Autodesk Inventor part; units mm, degrees
ref_plane "YZ Plane" through (0, 0, 0) normal (1, 0, 0) x (0, 1, 0)
ref_plane "XZ Plane" through (0, 0, 0) normal (0, 1, 0) x (-1, 0, 0)
ref_plane "XY Plane" through (0, 0, 0) normal (0, 0, 1) x (1, 0, 0)
sketch "Sketch1" plane through (0, 0, 0) normal (0, 1, 0) x (-1, 0, 0)
  line L0 (-3, 0) -> (-1.5, 2.5981)
  line L1 (-1.5, 2.5981) -> (1.5, 2.5981)
  line L2 (1.5, 2.5981) -> (3, 0)
  line L3 (3, 0) -> (1.5, -2.5981)
  line L4 (1.5, -2.5981) -> (-1.5, -2.5981)
  line L5 (-1.5, -2.5981) -> (-3, 0)
  point P0 (0, 0)
  point P1 (0, 0)
  dimension "d0" = 6
sketch "Sketch2" plane through (0, 0, 0) normal (0, 1, 0) x (-1, 0, 0)
  point P0 (0, 0)
extrude "Extrusion1" add sketch "Sketch1" along normal blind 25
sketch "Sketch3" plane through (0, 0, 0) normal (0, -1, 0) x (1, 0, 0)
  circle A0 centre (0, 0) radius 1.5
  dimension "d3" = 3
sketch "Sketch4" plane through (0, 25, 0) normal (0, 1, 0) x (1, 0, 0)
  circle A0 centre (0, 0) radius 1.5
  dimension "d4" = 3
extrude "Extrusion2" add sketch "Sketch3" along normal blind 8
extrude "Extrusion3" cut sketch "Sketch4" against normal blind 10
properties part number "Spacer25mm" material "Brass, Soft Yellow"
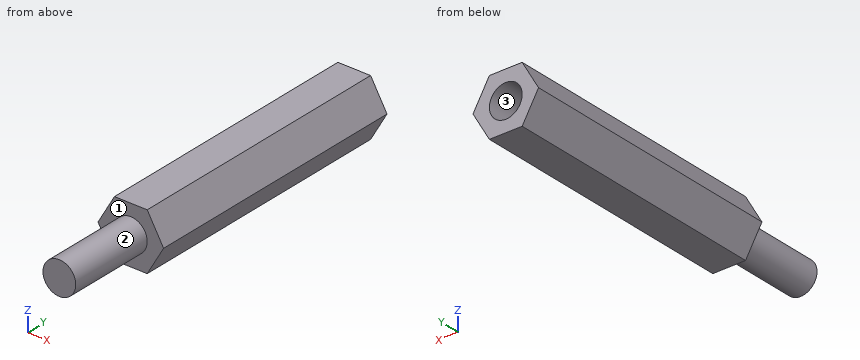
Model file for the job. Use its own axes, mm. Face numbers are marked on the shaded views. Give positions to 0.01 mm unless a question says otherwise; leave off trailing zeros. Loops run counter-clockwise (first coordinate to the right, second up) from the corner with the lowest first, then second, coordinate; pieces in that order, holes last. Notation, with made-up numbers: (80.5, 20) - (107.5, 20) arc R25 cw to (107.5, 37) - close; hole circle Ø10 at (33, -10.75). An arc over 180 degrees is marked (long way). One line per item, written item: value. Start each with the question number.
1. Pull direction Z, two halves, no side cores. Call the marked faces 1, 2 and 3: pulls with the +Z half, pulls with the -Z half, needs draft (parallel to the pull), parting line crosses it, or undercut.
2. Slice it at B-B (x = 0). List the corners of the cut face in (y, z).
3. Pin check, flat tips, straight feed: pin 1 (2 mm diameter, centred on y = 13.5, z = -2, fed in from +X); pin 2 (0.9 mm diameter, centred on x = -0.5, z = 0, fed in from +Y). Stop position of each tip, or through.
4. Probe L1, parallel to Z at x = 0, y = 17.25; L2, parallel to Y at x = -0.3, z = 0.35; L3, parallel to Y at x = 1.05, z = -2.2. List the from-to ranges inside material, lowest first. Write a range as from..to.
5. Slice it at D-D (z = 0.75). List the corners of the cut face in (x, y).
6. Slice it at C-C (y = 17.5). List the corners of the cut face in (x, z), plus the area to 3 significant figures.
7. Slice it at A-A (y = 9). List the corners of the cut face in (x, z), plus the area to 3 significant figures.
Solution:
1. face 1: needs draft
1. face 2: parting line crosses it
1. face 3: undercut
2. outline: (-8, -1.5) - (0, -1.5) - (0, -2.6) - (25, -2.6) - (25, -1.5) - (15, -1.5) - (15, 1.5) - (25, 1.5) - (25, 2.6) - (0, 2.6) - (0, 1.5) - (-8, 1.5) - close
3. pin 1: stops at x = 2.42
3. pin 2: stops at y = 15
4. L1: z = -2.6..-1.5, 1.5..2.6
4. L2: y = -8..15
4. L3: y = 0..25
5. outline: (-2.57, 0) - (-1.3, 0) - (-1.3, -8) - (1.3, -8) - (1.3, 0) - (2.57, 0) - (2.57, 25) - (1.3, 25) - (1.3, 15) - (-1.3, 15) - (-1.3, 25) - (-2.57, 25) - close
6. outline: (-3, 0) - (-1.5, -2.6) - (1.5, -2.6) - (3, 0) - (1.5, 2.6) - (-1.5, 2.6) - close; hole circle Ø3 at (0, 0)
6. area: 16.3 mm^2
7. outline: (-3, 0) - (-1.5, -2.6) - (1.5, -2.6) - (3, 0) - (1.5, 2.6) - (-1.5, 2.6) - close
7. area: 23.4 mm^2
